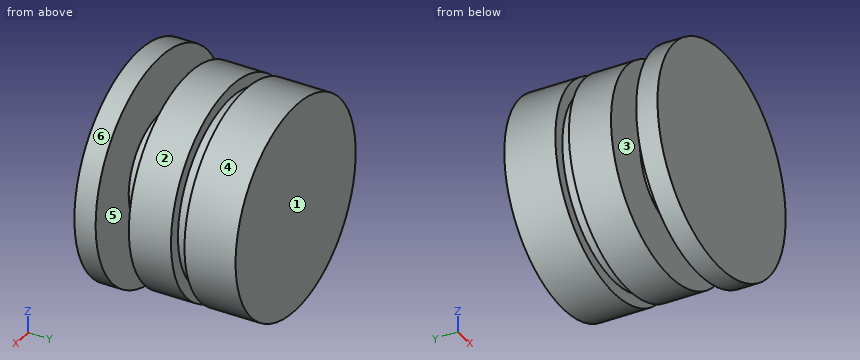
from build123d import *

# Parameters (mm, degrees)
MOUNTING_PLATE_SKETCH_R = 52.500000029
MOUNT_PLATE_DEPTH       = 10
SKETCH7_R               = 25.4
BOSS_EXTRUDE5_DEPTH     = 13.74902
SKETCH12_R              = 49.2125
BOSS_EXTRUDE6_DEPTH     = 50.23104
SKETCH15_W              = 5.715
SKETCH15_H              = 6.35


with BuildPart() as part:
    # Mounting Plate SKETCH → Mount Plate (new body)
    with BuildSketch(Plane(origin=(0, 0, 0), x_dir=(1, 0, 0), z_dir=(0, 1, 0))):
        with Locations(Location((0, 0, 0), (0, 0, 270))):
            Circle(MOUNTING_PLATE_SKETCH_R)
    extrude(amount=MOUNT_PLATE_DEPTH)

    # Sketch7 → Boss-Extrude5 (add)
    with BuildSketch(Plane(origin=(0, 10, 0), x_dir=(1, 0, 0), z_dir=(0, 1, 0))):
        with Locations(Location((0, 0, 0), (0, 0, 270))):
            Circle(SKETCH7_R)
    extrude(amount=BOSS_EXTRUDE5_DEPTH)

    # Sketch12 → Boss-Extrude6 (add)
    with BuildSketch(Plane(origin=(0, 23.74902, 0), x_dir=(1, 0, 0), z_dir=(0, 1, 0))):
        with Locations(Location((0, 0, 0), (0, 0, 270))):
            Circle(SKETCH12_R)
    extrude(amount=BOSS_EXTRUDE6_DEPTH)

    # Sketch15 → Cut-Revolve3 (revolve, cut)
    with BuildSketch(Plane(origin=(0, 0, 0), x_dir=(0, 0, -1), z_dir=(1, 0, 0)), mode=Mode.PRIVATE) as cut_revolve3_sk:
        with Locations((46.355, 46.76904)):
            Rectangle(SKETCH15_W, SKETCH15_H)
    revolve(cut_revolve3_sk.sketch.rotate(Axis((0, 0, 0), (0, -1, 0)), 180), axis=Axis((0, 0, 0), (0, -1, 0)), mode=Mode.SUBTRACT)


solid = part.part
Work out the finished part from the listing and answer in its coordinate system (mm). Face numbers are marked on the shaded views. A direction names the side the tool comes from. Round coordinates to 2 decimals unless told otherwise and drop trailing zeros. Write each loop counter-clockwise with the first axis right and the second up, starting at its lowest first coordinate (ties: lowest second). Pieces come first, ordered by that corner, then holes.
1) A cutting plane is placed at D-D (z = 0). Give the vertices of the cut face in (x, y), plus the area to 3 significant figures.
2) The mould has two halves that part along Y. Classify the marked faces 1, 2 and 3: pulls with the +Y half, pulls with the -Y half, needs draft (parallel to the pull), parting line crosses it, or undercut.
3) A cutting plane is placed at A-A (z = 42). Give the vertices of the cut face in (x, y), plus the area to 3 significant figures.
4) Straight lines are drawn through the part: line 1 (Y direction, x = -12.5, z = 47.5); line 2 (Y direction, x = 35, z = 2.5); line 3 (Y direction, x = -42.5, z = 29). For each, find the intervals that lie inside material, in ascending order.
5) A tool of negligible diameter and unlimited length cuts with its end or side. For the marked faces 4, 5 and 6, from which of +Z, -Z, +X, -X, +Y, -Y can it reach the whole face along a straight path? Write none if from no direction.
6) A cutting plane is placed at B-B (x = 32.5). Give the vertices of the cut face in (y, z).
7) Given pin 1 Ø1.5 at (y, z) = (46.5, -7.5) entering from +X; pin 2 Ø10 at (x, y) = (-41.5, 42) entering from -Z; pin 3 Ø3 at (y, z) = (31, -41) entering from +X, each flat-ended and moving along its own axis, determine where each tip first touches the part or whether it passes through.
8) A cutting plane is placed at C-C (x = 0). Give the vertices of the cut face in (y, z).
Completed:
1. outline: (-52.5, 0) - (52.5, 0) - (52.5, 10) - (25.4, 10) - (25.4, 23.75) - (49.21, 23.75) - (49.21, 43.59) - (43.5, 43.59) - (43.5, 49.94) - (49.21, 49.94) - (49.21, 73.98) - (-49.21, 73.98) - (-49.21, 49.94) - (-43.5, 49.94) - (-43.5, 43.59) - (-49.21, 43.59) - (-49.21, 23.75) - (-25.4, 23.75) - (-25.4, 10) - (-52.5, 10) - close
1. area: 6,620 mm2
2. face 1: pulls with the +Y half
2. face 2: needs draft
2. face 3: undercut
3. outline: (-31.5, 0) - (31.5, 0) - (31.5, 10) - (-31.5, 10) - close; (-25.65, 23.75) - (25.65, 23.75) - (25.65, 43.59) - (11.32, 43.59) - (11.32, 49.94) - (25.65, 49.94) - (25.65, 73.98) - (-25.65, 73.98) - (-25.65, 49.94) - (-11.32, 49.94) - (-11.32, 43.59) - (-25.65, 43.59) - close
3. area: 3,020 mm2
4. line 1: y = 0 to 10, 23.75 to 43.59, 49.94 to 73.98
4. line 2: y = 0 to 10, 23.75 to 73.98
4. line 3: y = 0 to 10
5. face 4: +Y
5. face 5: none
5. face 6: +Y, -Y
6. outline: (0, -41.23) - (10, -41.23) - (10, 41.23) - (0, 41.23) - close; (23.75, -36.95) - (43.59, -36.95) - (43.59, -28.91) - (49.94, -28.91) - (49.94, -36.95) - (73.98, -36.95) - (73.98, 36.95) - (49.94, 36.95) - (49.94, 28.91) - (43.59, 28.91) - (43.59, 36.95) - (23.75, 36.95) - close
7. pin 1: stops at x = 42.97
7. pin 2: stops at z = -33.01
7. pin 3: stops at x = 29.35
8. outline: (0, -52.5) - (10, -52.5) - (10, -25.4) - (23.75, -25.4) - (23.75, -49.21) - (43.59, -49.21) - (43.59, -43.5) - (49.94, -43.5) - (49.94, -49.21) - (73.98, -49.21) - (73.98, 49.21) - (49.94, 49.21) - (49.94, 43.5) - (43.59, 43.5) - (43.59, 49.21) - (23.75, 49.21) - (23.75, 25.4) - (10, 25.4) - (10, 52.5) - (0, 52.5) - close
